```python
from build123d import *

# Parameters (mm, degrees)
BOSS_EXTRU_1_DEPTH      = 57
ESQUISSE2_R             = 2
ENL_V_MAT_EXTRU_1_DEPTH = 50
ESQUISSE3_R             = 1.5
ENL_V_MAT_EXTRU_2_DEPTH = 50


with BuildPart() as part:
    # Esquisse1 → Boss.-Extru.1 (new body)
    with BuildSketch(Plane(origin=(0, 0, 0), x_dir=(1, 0, 0), z_dir=(0, 1, 0))):
        Polygon((-11, 8.5), (-11, -1.5), (9, -1.5), (9, -0.5), (-10, -0.5), (-10, 8.5), align=None)
    extrude(amount=BOSS_EXTRU_1_DEPTH)

    # Esquisse2 → Enlèv. mat.-Extru.1 (cut)
    with BuildSketch(Plane.ZY.offset(11)):
        with Locations((-3.5, 52.14)):
            Circle(ESQUISSE2_R)
        with Locations((-3.5, 5)):
            Circle(ESQUISSE2_R)
    extrude(amount=-ENL_V_MAT_EXTRU_1_DEPTH, mode=Mode.SUBTRACT)

    # Esquisse3 → Enlèv. mat.-Extru.2 (cut)
    with BuildSketch(Plane(origin=(0, 0, 0.5), x_dir=(-1, 0, 0), z_dir=(0, 0, -1))):
        with Locations((1, 52)):
            Circle(ESQUISSE3_R)
        with Locations((1, 5)):
            Circle(ESQUISSE3_R)
        Polygon((2, 57), (-9, 46), (-9, 57), align=None)
        Polygon((-9, 0), (-9, 11), (2, 0), align=None)
    extrude(amount=-ENL_V_MAT_EXTRU_2_DEPTH, mode=Mode.SUBTRACT)


solid = part.part
```
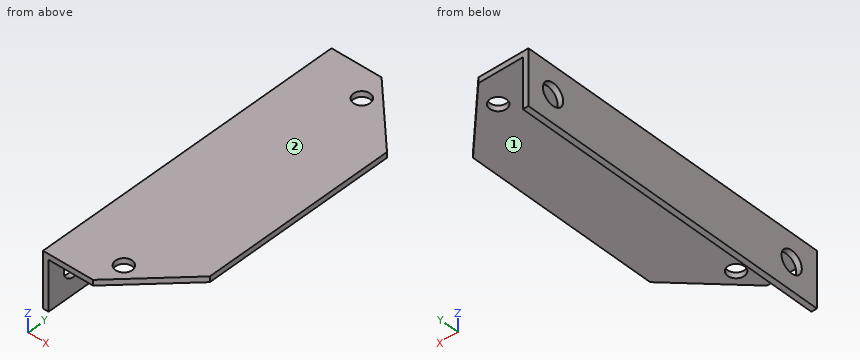
Can you work these out from the model? Positions are in its coordinate system, mm. Face numbers are marked on the shaded views. A direction names the side the tool comes from. Coordinates: 2 decimals unless noted, no trailing zeros. Order: outer loops, then holes, each group sorted by start corner. A loop starts at its lowest first (then second) coordinate and runs counter-clockwise, first axis right, second up. Notation, with made-up numbers: (-8.75, 30) -> (50.25, 30) arc R13 cw to (50.25, 51) -> close; hole circle Ø5 at (-3, 3). An arc over 180 degrees is marked (long way). Write each question's results on one line, items separated by ' | '.
Item 1: I'm going to push flat-ended pins straight in: pin 1 Ø5 at (x, y) = (-1.5, 14) entering from -Z; pin 2 Ø2 at (y, z) = (10, -3) entering from +X; pin 3 Ø2 at (x, z) = (4, -1) entering from -Y. Where does each tip first touch, or does it pass through?
Results are:
pin 1: z = 0.5 | pin 2: x = -10 | pin 3: through
Item 2: I want a section at B-B, the plane z = -3.5. Write out the boundary of the cut face in (x, y), then the cut area to 3 significant figures.
Results are:
outline: (-11, 0) -> (-10, 0) -> (-10, 3) -> (-11, 3) -> close; (-11, 7) -> (-10, 7) -> (-10, 50.14) -> (-11, 50.14) -> close; (-11, 54.14) -> (-10, 54.14) -> (-10, 57) -> (-11, 57) -> close | area: 49.0 mm²
Item 3: I want a section at A-A, the plane x = -1. Write out the boundary of the cut face in (y, z), then the cut area to 3 significant figures.
Results are:
outline: (1, 0.5) -> (3.5, 0.5) -> (3.5, 1.5) -> (1, 1.5) -> close; (6.5, 0.5) -> (50.5, 0.5) -> (50.5, 1.5) -> (6.5, 1.5) -> close; (53.5, 0.5) -> (56, 0.5) -> (56, 1.5) -> (53.5, 1.5) -> close | area: 49.0 mm²
Item 4: I want a section at C-C, the plane y = 5. Write out the boundary of the cut face in (x, z), then the cut area to 3 significant figures.
Results are:
outline: (-11, -8.5) -> (-10, -8.5) -> (-10, -5.5) -> (-11, -5.5) -> close; (-11, -1.5) -> (-10, -1.5) -> (-10, 0.5) -> (-2.5, 0.5) -> (-2.5, 1.5) -> (-11, 1.5) -> close; (0.5, 0.5) -> (3, 0.5) -> (3, 1.5) -> (0.5, 1.5) -> close | area: 16.0 mm²
Item 5: I want a section at D-D, the plane y = 23. Write out the boundary of the cut face in (x, z), then the cut area to 3 significant figures.
Results are:
outline: (-11, -8.5) -> (-10, -8.5) -> (-10, 0.5) -> (9, 0.5) -> (9, 1.5) -> (-11, 1.5) -> close | area: 29.0 mm²
Item 6: If I drill on line 1 along Y through (x, z) = (-10.8, -3.5); line 2 along Y through (x, z) = (-1, 1.15); line 3 along Z through (x, y) = (3.5, 24), over which ranges is the centre line in solid material (lowest first)?
Results are:
line 1: 0 to 3, 7 to 50.14, 54.14 to 57 | line 2: 1 to 3.5, 6.5 to 50.5, 53.5 to 56 | line 3: 0.5 to 1.5
Item 7: Which directions (+Z, -Z, +X, -X, +Y, -Y) give clear straight access to the entire face, cutting with the end or side of a thin tool? Please do the marked faces 1 and 2.
Results are:
face 1: -Z, +X, +Y, -Y | face 2: +Z, +X, -X, +Y, -Y
